Work out the finished part from the listing and answer in its coordinate system (mm). Round coordinates to 2 decimals unless told otherwise and drop trailing zeros. Loops run counter-clockwise (first coordinate to the right, second up) from the corner with the lowest first, then second, coordinate; pieces in that order, holes last. Notation, with made-up numbers: (38.25, 11) -> (48.25, 11) arc R16 cw to (48.25, 18) -> close; hole circle Ø9 at (-10, 78.5). An arc over 180 degrees is marked (long way). Use one line per item in the form item = value.
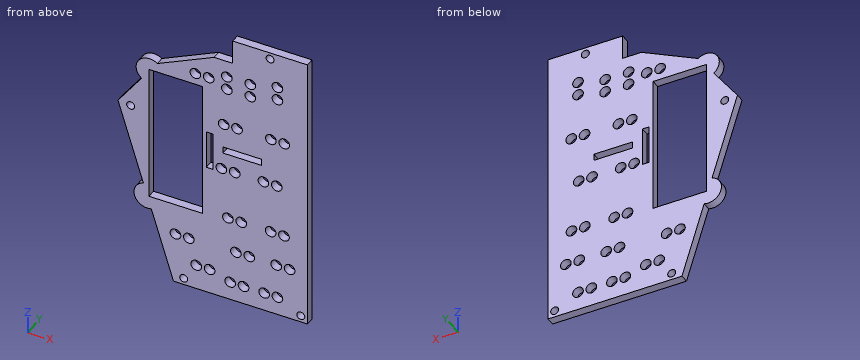
```python
from build123d import *

# Parameters (mm, degrees)
SKETCH1_R           = 1.5
SKETCH1_R_2         = 2
SKETCH1_W           = 2.5
SKETCH1_H           = 14.5
SKETCH1_W_2         = 14.5
SKETCH1_H_2         = 2.5
SKETCH1_W_3         = 20
SKETCH1_H_3         = 52
BOSS_EXTRUDE1_DEPTH = 3.175


with BuildPart() as part:
    # Sketch1 → Boss-Extrude1 (new body)
    with BuildSketch(Plane(origin=(0, 0, 0), x_dir=(1, 0, 0), z_dir=(0, 1, 0))):
        with BuildLine():
            Line((-22.047586286, 28.724844999), (28.152410312, 28.724844999))
            Line((28.152410312, 28.724844999), (28.152410312, -68.278843574))
            Line((28.152410312, -68.278843574), (28.152410312, -77.482069575))
            Line((28.152410312, -77.482069575), (0.152410312, -77.482069575))
            Line((0.152410312, -77.482069575), (0.152410312, -68.337119167))
            Line((0.152410312, -68.337119167), (-6.847541173, -68.337119167))
            Line((-6.847541173, -68.337119167), (-28.095254294, -58.371916125))
            ThreePointArc((-28.095254294, -58.371916125), (-35.084160474, -57.28326894), (-33.991325412, -50.295016382))
            Line((-33.991325412, -50.295016382), (-42.847532209, -38.188499756))
            Line((-42.847532209, -38.188499756), (-33.328350902, -7.56533069))
            ThreePointArc((-33.328350902, -7.56533069), (-36.624195189, -1.304825925), (-30.359969494, 1.9839407))
            Line((-30.359969494, 1.9839407), (-22.047586286, 28.724844999))
        make_face()
        with Locations((25.652410312, 26.224844999)):
            Circle(SKETCH1_R, mode=Mode.SUBTRACT)
        with Locations((-38.087063045, -37.694179546)):
            Circle(SKETCH1_R, mode=Mode.SUBTRACT)
        with Locations((-18.207043121, 26.221156426)):
            Circle(SKETCH1_R, mode=Mode.SUBTRACT)
        with Locations((16.902410312, 21.724844999)):
            Circle(SKETCH1_R_2, mode=Mode.SUBTRACT)
        with Locations((11.902410312, 21.724844999)):
            Circle(SKETCH1_R_2, mode=Mode.SUBTRACT)
        with Locations((4.202410312, 21.724844999)):
            Circle(SKETCH1_R_2, mode=Mode.SUBTRACT)
        with Locations((-0.797589688, 21.724844999)):
            Circle(SKETCH1_R_2, mode=Mode.SUBTRACT)
        with Locations((-8.518099948, 19.221156426)):
            Circle(SKETCH1_R_2, mode=Mode.SUBTRACT)
        with Locations((-13.518099948, 19.221156426)):
            Circle(SKETCH1_R_2, mode=Mode.SUBTRACT)
        with Locations((-16.301455712, 9.146912193)):
            Circle(SKETCH1_R_2, mode=Mode.SUBTRACT)
        with Locations((-21.301455712, 9.146912193)):
            Circle(SKETCH1_R_2, mode=Mode.SUBTRACT)
        with Locations((-2.047589688, -61.948843574)):
            Circle(SKETCH1_R_2, mode=Mode.SUBTRACT)
        with Locations((-2.047589688, -56.948843574)):
            Circle(SKETCH1_R_2, mode=Mode.SUBTRACT)
        with Locations((6.752410312, -61.948843574)):
            Circle(SKETCH1_R_2, mode=Mode.SUBTRACT)
        with Locations((6.752410312, -56.948843574)):
            Circle(SKETCH1_R_2, mode=Mode.SUBTRACT)
        with Locations((-8.847589688, -59.278843574)):
            Circle(SKETCH1_R_2, mode=Mode.SUBTRACT)
        with Locations((-13.847589688, -59.278843574)):
            Circle(SKETCH1_R_2, mode=Mode.SUBTRACT)
        with Locations((21.452410312, 8.724844999)):
            Circle(SKETCH1_R_2, mode=Mode.SUBTRACT)
        with Locations((16.452410312, 8.724844999)):
            Circle(SKETCH1_R_2, mode=Mode.SUBTRACT)
        with Locations((6.352410312, 8.724844999)):
            Circle(SKETCH1_R_2, mode=Mode.SUBTRACT)
        with Locations((1.352410312, 8.724844999)):
            Circle(SKETCH1_R_2, mode=Mode.SUBTRACT)
        with Locations((14.352410312, -4.275155001)):
            Circle(SKETCH1_R_2, mode=Mode.SUBTRACT)
        with Locations((19.352410312, -4.275155001)):
            Circle(SKETCH1_R_2, mode=Mode.SUBTRACT)
        with Locations((3.352410312, -4.275155001)):
            Circle(SKETCH1_R_2, mode=Mode.SUBTRACT)
        with Locations((-1.647589688, -4.275155001)):
            Circle(SKETCH1_R_2, mode=Mode.SUBTRACT)
        with Locations((16.652410312, -23.778843574)):
            Circle(SKETCH1_R_2, mode=Mode.SUBTRACT)
        with Locations((11.652410312, -23.778843574)):
            Circle(SKETCH1_R_2, mode=Mode.SUBTRACT)
        with Locations((0.902410312, -23.778843574)):
            Circle(SKETCH1_R_2, mode=Mode.SUBTRACT)
        with Locations((-4.097589688, -23.778843574)):
            Circle(SKETCH1_R_2, mode=Mode.SUBTRACT)
        with Locations((19.452410312, -42.075155001)):
            Circle(SKETCH1_R_2, mode=Mode.SUBTRACT)
        with Locations((14.452410312, -42.075155001)):
            Circle(SKETCH1_R_2, mode=Mode.SUBTRACT)
        with Locations((1.752410312, -42.075155001)):
            Circle(SKETCH1_R_2, mode=Mode.SUBTRACT)
        with Locations((-3.247589688, -42.075155001)):
            Circle(SKETCH1_R_2, mode=Mode.SUBTRACT)
        with Locations((16.902410312, -59.278843574)):
            Circle(SKETCH1_R_2, mode=Mode.SUBTRACT)
        with Locations((16.902410312, -64.278843574)):
            Circle(SKETCH1_R_2, mode=Mode.SUBTRACT)
        with Locations((14.152410312, -74.982069575)):
            Circle(SKETCH1_R, mode=Mode.SUBTRACT)
        with Locations((-8.497589688, -29.525155001)):
            Rectangle(SKETCH1_W, SKETCH1_H, mode=Mode.SUBTRACT)
        with Locations((3.702410312, -31.528843574)):
            Rectangle(SKETCH1_W_2, SKETCH1_H_2, mode=Mode.SUBTRACT)
        with Locations((-21.247589688, -28.865155001)):
            Rectangle(SKETCH1_W_3, SKETCH1_H_3, mode=Mode.SUBTRACT)
    extrude(amount=BOSS_EXTRUDE1_DEPTH)


solid = part.part
```
(1) Consider L1, parallel to X at y = 2.05, z = 39; L2, parallel to Z at x = -9, y = 2.8; L3, parallel to X at y = 0.8, z = 63.5. Determine where each line is inside the solid, lowest interval first.
Completed:
L1 = -42.25 to -38.83, -37.35 to -31.25, -11.25 to 28.15
L2 = -28.72 to -21.16, -17.28 to 22.28, 36.78 to 57.28, 61.27 to 67.33
L3 = -17.16 to -3.31, -0.79 to 5.49, 8.01 to 15.06, 18.74 to 28.15
(2) Find section C-C, the plane y = 1.7. State how many separate pieces and enclosed holes the cut face has, then the cut area to 3 significant figures.
Completed:
separate_pieces = 1
enclosed_holes = 39
area = 4,590 mm2
(3) Find section B-B, the plane z = 13.5. Write down the section's boundary in (x, y) (3 decimals), then the cut area to 3 significant figures.
Completed:
outline = (-35.173, 0) -> (-31.248, 0) -> (-31.248, 3.175) -> (-35.173, 3.175) -> close; (-11.248, 0) -> (28.152, 0) -> (28.152, 3.175) -> (-11.248, 3.175) -> close
area = 138 mm2
(4) Find section A-A, the plane x = -38. Write down the section's boundary in (y, z) (3 decimals), then the cut area to 3 significant figures.
Completed:
outline = (0, 22.594) -> (3.175, 22.594) -> (3.175, 36.197) -> (0, 36.197) -> close; (0, 39.192) -> (3.175, 39.192) -> (3.175, 44.815) -> (0, 44.815) -> close
area = 61.0 mm2
(5) Find section D-D, the plane z = -13. Write down the section's boundary in (x, y) (3 decimals).
Completed:
outline = (-26.936, 0) -> (28.152, 0) -> (28.152, 3.175) -> (-26.936, 3.175) -> close
(6) Given P1, Ø1, axis at x = -4, y = 2, coming from the +Z side; P2, Ø1.6, axis at y = 2.5, z = 72.5, coming from the -X side, each flat-ended and moving along its own axis, determine where each tip first touches the part or whether it passes through.
Completed:
P1 = 68.34
P2 = 0.15
